Input: dimensioned drawing with shaded views. Units: mm. Origin: part minimum x, y, z. Give positions to 0.01 mm unless a question says otherwise; leave off trailing zeros. Write each loop counter-clockwise with the first axis right and the second up, starting at its lowest first coordinate (ties: lowest second). Pieces come first, ordered by that corner, then holes.
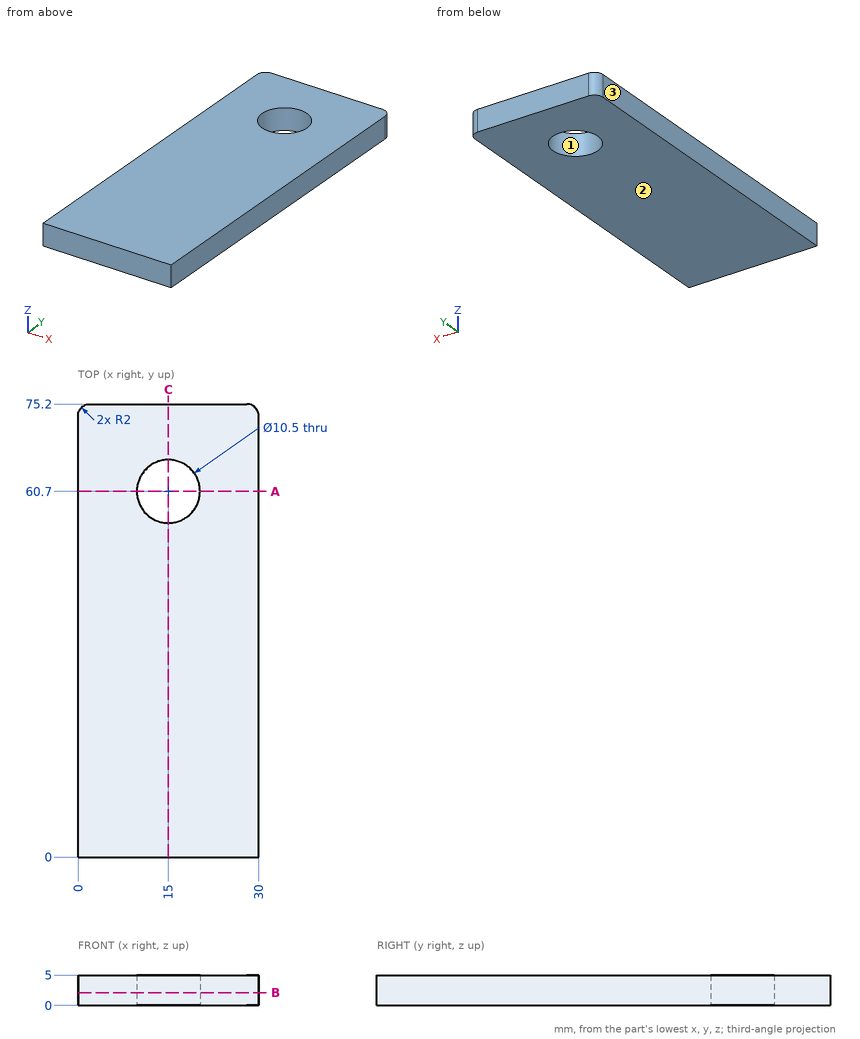
Item 1: Section A-A, the plane y = 60.7. Return the cut outline in (x, z), plus the area to 3 significant figures.
Found:
outline: (0, 0) - (9.75, 0) - (9.75, 5) - (0, 5) - close; (20.25, 0) - (30, 0) - (30, 5) - (20.25, 5) - close
area: 97.5 mm2
Item 2: Section C-C, the plane x = 15. Return the cut outline in (y, z).
Found:
outline: (0, 0) - (55.45, 0) - (55.45, 5) - (0, 5) - close; (65.95, 0) - (75.2, 0) - (75.2, 5) - (65.95, 5) - close
Item 3: Pull-direction query (X, two-part tool) for the marked faces 1, 2 and 3; classes: +X half, -X half, draft (parallel to the pull), parting line (faces both ways), or undercut.
Found:
face 1: undercut
face 2: draft
face 3: -X half
Item 4: Line query: L1, parallel to Y at x = 15, z = 2.6; L2, parallel to Y at x = 12.5, z = 1.6. Output: solid intervals per line, ascending.
Found:
L1: y = 0 to 55.45, 65.95 to 75.2
L2: y = 0 to 56.08, 65.32 to 75.2
Item 5: Section B-B, the plane z = 2.1. Return the cut outline in (x, y).
Found:
outline: (0, 0) - (30, 0) - (30, 73.2) arc R2 ccw to (28, 75.2) - (2, 75.2) arc R2 ccw to (0, 73.2) - close; hole circle Ø10.5 at (15, 60.7)
